CAD build for the part. Positions are in the model's coordinates, mm. A direction names the side the tool comes from. Give positions to 0.01 mm unless a question says otherwise; leave off trailing zeros. Order: outer loops, then holes, each group sorted by start corner. A loop starts at its lowest first (then second) coordinate and runs counter-clockwise, first axis right, second up. Notation, with made-up numbers: (5, -36) -> (50, -36) arc R27 ccw to (50, -10) -> close; hole circle Ø5 at (83.25, 61). An arc over 180 degrees is marked (long way). Use one line per item in the form item = value. Start each with the question number.
1) Cut at C-C, the plane x = -61. Give the cut face in (y, z), and give its area (3 significant figures).
2) Cut at A-A, the plane y = -467.75. Give the cut face in (x, z).
3) Probe line 1 (Y direction, x = -30, z = 1.3); line 2 (Y direction, x = 0, z = -6); line 3 (Z direction, x = -84, y = 17). List the from-to ranges inside material, lowest first.
4) Tool access for faces 1 (the face through (73.713, 0.352, 1.479)), 2 (the face through (9, -479, 0)): list every direction of +Z, -Z, +X, -X, +Y, -Y with a clear straight run to the whole face (end or side of a thin tool).
5) Mould opens along X. For faces 3 (the face through (-1.653, -455.158, -9.86)), 4 (the face through (91.445, 75.979, 1.479)), 5 (the face through (0, 0, -10)), 6 (the face through (-91.445, -75.979, 1.479)) say: pulls with the +X half, pulls with the -X half, needs draft (parallel to the pull), parting line crosses it, or undercut.
6) Cut at B-B, the plane z = -4.75. Give the cut face in (x, y).
7) Drop flat-ended pins along their axis: P1, Ø4, axis at y = -521, z = -2.5, coming from the +X side; P2, Ø6, axis at y = -699.5, z = -11, coming from the -X side; P3, Ø1.5, axis at x = -27.5, z = 2, coming from the -Y side. Give the stop position or say it passes through.
from build123d import *

# Parameters (mm, degrees)
CROQUIS1_R              = 8
CROQUIS1_R_2            = 4
SALIENTE_EXTRUIR1_DEPTH = 3
CROQUIS2_W              = 40
CROQUIS2_H              = 885
CROQUIS2_R              = 12.7
SALIENTE_EXTRUIR2_DEPTH = 20


with BuildPart() as part:
    # Croquis1 → Saliente-Extruir1 (new body)
    with BuildSketch(Plane.XY):
        with BuildLine():
            Line((70, 85), (-70, 85))
            ThreePointArc((-70, 85), (-91.213203436, 76.213203436), (-100, 55))
            Line((-100, 55), (-100, -55))
            ThreePointArc((-100, -55), (-91.213203436, -76.213203436), (-70, -85))
            Line((-70, -85), (70, -85))
            ThreePointArc((70, -85), (91.213203436, -76.213203436), (100, -55))
            Line((100, -55), (100, 55))
            ThreePointArc((100, 55), (91.213203436, 76.213203436), (70, 85))
        make_face()
        with Locations((-81.705, 0)):
            Circle(CROQUIS1_R, mode=Mode.SUBTRACT)
        with Locations((81.705, 0)):
            Circle(CROQUIS1_R, mode=Mode.SUBTRACT)
        with Locations((0, 70.6)):
            Circle(CROQUIS1_R_2, mode=Mode.SUBTRACT)
        with Locations((0, -70.6)):
            Circle(CROQUIS1_R_2, mode=Mode.SUBTRACT)
        with Locations((-30, 70.6)):
            Circle(CROQUIS1_R_2, mode=Mode.SUBTRACT)
        with Locations((30, 70.6)):
            Circle(CROQUIS1_R_2, mode=Mode.SUBTRACT)
        with Locations((-30, -70.6)):
            Circle(CROQUIS1_R_2, mode=Mode.SUBTRACT)
        with Locations((30, -70.6)):
            Circle(CROQUIS1_R_2, mode=Mode.SUBTRACT)
    extrude(amount=SALIENTE_EXTRUIR1_DEPTH)

    # Croquis2 → Saliente-Extruir2 (add)
    with BuildSketch(Plane.XY):
        with Locations((0, -442.5)):
            Rectangle(CROQUIS2_W, CROQUIS2_H)
        with Locations((0, -467.75)):
            Circle(CROQUIS2_R, mode=Mode.SUBTRACT)
    extrude(amount=-SALIENTE_EXTRUIR2_DEPTH)


solid = part.part
Result:
q1.outline = (-85, 0) -> (85, 0) -> (85, 3) -> (-85, 3) -> close
q1.area = 510 mm²
q2.outline = (-20, -20) -> (-12.7, -20) -> (-12.7, 0) -> (-20, 0) -> close; (12.7, -20) -> (20, -20) -> (20, 0) -> (12.7, 0) -> close
q3.line_1 = -85 to -74.6, -66.6 to 66.6, 74.6 to 85
q3.line_2 = -885 to -480.45, -455.05 to 0
q3.line_3 = 0 to 3
q4.face_1 = +Z, -Z
q4.face_2 = +Z, +X, -X, -Y
q5.face_3 = undercut
q5.face_4 = pulls with the +X half
q5.face_5 = needs draft
q5.face_6 = pulls with the -X half
q6.outline = (-20, -885) -> (20, -885) -> (20, 0) -> (-20, 0) -> close; hole circle Ø25.4 at (0, -467.75)
q7.P1 = 20
q7.P2 = -20
q7.P3 = -85
